Autodesk Inventor part; units mm, degrees
ref_plane "YZ Plane" through (0, 0, 0) normal (1, 0, 0) x (0, 1, 0)
ref_plane "XZ Plane" through (0, 0, 0) normal (0, 1, 0) x (-1, 0, 0)
ref_plane "XY Plane" through (0, 0, 0) normal (0, 0, 1) x (1, 0, 0)
sketch "Sketch1" plane through (0, 0, 0) normal (0, 1, 0) x (-1, 0, 0)
  line L0 (0, 0) -> (-15, 0)
  line L1 (-15, 0) -> (-15, -10)
  line L2 (-15, -10) -> (0, -10)
  line L3 (0, -10) -> (0, 0)
  dimension "d0" = 10
  dimension "d1" = 15
extrude "Extrusion1" add sketch "Sketch1" along normal blind 10
sketch "Sketch2" plane through (0, 10, 0) normal (0, 1, 0) x (1, 0, 0)
  line L0 (0.0305, 1.2348) -> (7.5305, 1.2348)
  line L1 (7.5305, 1.2348) -> (7.5305, 6.2348)
  line L2 (7.5305, 6.2348) -> (0.0305, 6.2348)
  line L3 (0.0305, 6.2348) -> (0.0305, 1.2348)
  point P0 (0, 0)
  dimension "d4" = 5
  dimension "d5" = 7.5
revolve "Revolution1" add sketch "Sketch2" angle 90 about axis through (0.0305, 10, -1.2348) along (1, 0, 0)
fillet "Fillet1" radius 2 3 edges at (7.5, 10, 0) (15, 10, -5) (15, 5, 0)
sketch "Sketch3" plane through (0, 0, 0) normal (0, 0, 1) x (1, 0, 0)
  point P0 (0, 0)
  point P1 (5.4835, 3.5664)
hole "Hole1" at (5.4835, 3.5664, 0) direction (0, 0, -1) diameter 3 end through all
properties part number "TEAM4788-001-Test-Part"
Source: CAD feature listing. Evaluate the final solid. Frame: model axes, mm. A direction names the side the tool comes from. Round coordinates to 2 decimals unless told otherwise and drop trailing zeros. Loops run counter-clockwise (first coordinate to the right, second up) from the corner with the lowest first, then second, coordinate; pieces in that order, holes last. Notation, with made-up numbers: (51.5, 16.5) - (105.5, 16.5) arc R20 ccw to (105.5, 25.5) - close; hole circle Ø8 at (-26.75, 45.25). An arc over 180 degrees is marked (long way). Write item = value, one per line. Start each with the question number.
(1) Section query B-B, the plane y = 3. Output: boundary loops of the cut face in (x, z), plus the area to 3 significant figures.
(2) Pull-direction query (X, two-part tool) for faces 3 (the face through (4.5, 4.7, -5.1)), 4 (the face through (8, 5, -10)), 5 (the face through (0, 5, -5)), 6 (the face through (7.53, 12, -3)); classes: +X half, -X half, draft (parallel to the pull), parting line (faces both ways), or undercut.
(3) Ray query, line 1 along Y through (x, z) = (5.5, -7.25); line 2 along Y through (x, z) = (6, -7.75); line 3 along Y through (x, z) = (8.25, -8.25). Return the intervals inside material, ascending. Write a range as from..to.
(4) Set-up query: faces 1 (the face through (4, 12, -1.235)), 2 (the face through (8, 0, -5)). Return all of +Z, -Z, +X, -X, +Y, -Y with unobstructed straight access to the full face (end or side cutting, diameter ignored); none if empty.
(5) Section query D-D, the plane x = 3.25. Output: boundary loops of the cut face in (y, z).
(6) Section query A-A, the plane x = 6.75. Output: boundary loops of the cut face in (y, z), plus the area to 3 significant figures.
(7) Pin query (flat end, axial travel): pin 1 (5.5 mm diameter, centred on y = 13, z = -4, fed in from +X); pin 2 (2.5 mm diameter, centred on y = 13, z = -4.5, fed in from -X); pin 3 (5.5 mm diameter, centred on x = 5, y = 12, fed in from +Z). Return the tip coordinate at first contact, or that it passes through.
Conclusion:
q1.outline = (0, -10) - (4.09, -10) - (4.09, 0) - (0, 0) - close; (6.87, -10) - (15, -10) - (15, -2) arc R2 ccw to (13, 0) - (6.87, 0) - close
q1.area = 121 mm2
q2.face_3 = undercut
q2.face_4 = draft
q2.face_5 = -X half
q2.face_6 = +X half
q3.line_1 = 0..2.07, 5.07..10
q3.line_2 = 0..2.16, 4.97..10
q3.line_3 = 0..10
q4.face_1 = +Z, +X, -X, +Y
q4.face_2 = +Z, -Z, +X, -X, -Y
q5.outline = (0, -10) - (10, -10) - (10, -6.23) arc R5 ccw to (15, -1.23) - (9.85, -1.23) arc R2 ccw to (8, 0) - (0, 0) - close
q6.outline = (0, -10) - (2.76, -10) - (2.76, 0) - (0, 0) - close; (4.37, -10) - (10, -10) - (10, -6.23) arc R5 ccw to (15, -1.23) - (9.85, -1.23) arc R2 ccw to (8, 0) - (4.37, 0) - close
q6.area = 103 mm2
q7.pin_1 = 7.53
q7.pin_2 = 0.03
q7.pin_3 = -0.44
